Read the model definition and answer for the solid it produces. Units are mm, in the model's axes. A direction names the side the tool comes from. Give positions to 0.01 mm unless a question says otherwise; leave off trailing zeros. Write each loop counter-clockwise with the first axis right and the second up, starting at its lowest first coordinate (ties: lowest second). Pieces come first, ordered by that corner, then holes. Notation, with made-up numbers: (81.5, -16.5) - (118.5, -16.5) arc R26 ccw to (118.5, 8.5) - close; hole circle Ø8 at (82, 79.25). An arc over 180 degrees is marked (long way). Answer as CSV lines item,"result".
Autodesk Inventor part; units mm, degrees
ref_plane "YZ Plane" through (0, 0, 0) normal (1, 0, 0) x (0, 1, 0)
ref_plane "XZ Plane" through (0, 0, 0) normal (0, 1, 0) x (-1, 0, 0)
ref_plane "XY Plane" through (0, 0, 0) normal (0, 0, 1) x (1, 0, 0)
sketch "Szkic1" plane through (0, 0, 0) normal (0, 1, 0) x (-1, 0, 0)
  line L0 (8.460922, -2.595157) -> (8.460922, -202.595157)
  line L1 (8.460922, -202.595157) -> (-191.539078, -202.595157)
  line L2 (8.460922, -2.595157) -> (-191.539078, -2.595157)
  line L3 (8.460922, -2.595157) -> (208.460922, -2.595157) construction
  arc A0 (-191.539078, -2.595157) -> (-191.539078, -202.595157) centre (-145.713321, -102.595157) ccw
  line L4 (8.460922, -102.595157) -> (43.460922, -102.595157) construction
  circle A1 centre (-26.539078, -102.595157) radius 10
  point P0 (0, 0)
  dimension "d0" = 200
  dimension "d1" = 200
  dimension "d2" = 90
  dimension "d4" = 200
  dimension "d5" = 180
  dimension "d6" = 110
  dimension "d10" = 20
extrude "Wyciągnięcie proste1" add sketch "Szkic1" along normal blind 74.5
sketch "Szkic2" plane through (0, 74.5, 0) normal (0, 1, 0) x (1, 0, 0)
  circle A0 centre (107.96185, 52.890403) radius 34.51232
  circle A1 centre (113.959733, 99.782925) radius 48.14156
  point P0 (0, 0)
sketch "Szkic2 outline for Wyciągnięcie proste2" plane through (0, 74.5, 0) normal (0, 1, 0) x (1, 0, 0)
  circle A0 centre (113.959733, 99.782925) radius 48.14156
extrude "Wyciągnięcie proste2" add sketch "Szkic2 outline for Wyciągnięcie proste2" along normal blind 74.5 draft -10
hole "Otwór1" at (114.99325, 149, -100.1379) direction (0, -1, 0) diameter 25.75 end through all
(1) For faces 5 (the flat face through (90, 37, -202.595)), 6 (the flat face through (96, 74.5, -146)), determine the directions among +Z, -Z, +X, -X, +Y, -Y from which every point of the face is accessible in a straight line to the end or side of a thin tool.
Worked out:
face 5,"-Z, +X, -X, +Y, -Y"
face 6,"+Y"
(2) A cutting plane is placed at B-B (y = 80.5). Write down the section's boundary in (x, z) (3 decimals).
Worked out:
outline,"circle Ø94.167 at (113.96, -99.783); hole circle Ø25.75 at (114.993, -100.138)"
(3) Find the intervals of material crossed by L1, parallel to Y at x = 225.5, z = -138; L2, parallel to X at y = 30, z = -109.5; L3, parallel to Z at x = 123, y = 81.5, in increasing order.
Worked out:
L1,"y = 0 to 74.5"
L2,"x = -8.46 to 19.31, 33.77 to 106.15, 123.83 to 255.5"
L3,"z = -145.81 to -110.22, -90.06 to -53.76"
(4) A cutting plane is placed at D-D (z = -30). Write down the section's boundary in (x, y).
Worked out:
outline,"(-8.46, 0) - (228.36, 0) - (228.36, 74.5) - (-8.46, 74.5) - close"
(5) Each of these flat-tipped pins is pushed along its axis until it touches: P1, Ø10, axis at x = 182.5, z = -78.5, coming from the +Y side; P2, Ø12, axis at y = 27, z = -112.5, coming from the +X side; P3, Ø3, axis at x = 199.5, y = 34.5, coming from the -Z side. Where does it stop, or does it pass through?
Worked out:
P1,"stops at y = 74.5"
P2,"stops at x = 255.64"
P3,"stops at z = -199.37"
(6) A cutting plane is placed at A-A (x = 58). Write down the section's boundary in (y, z).
Worked out:
outline,"(0, -202.6) - (74.5, -202.6) - (74.5, -2.6) - (0, -2.6) - close"
(7) The mould has two halves that part along X. Classify faces 1 (the flat face through (129, 149, -100)), 2 (the cylindrical face through (17.3, 36.73, -98.77)), 3 (the cylindrical face through (106.292, 73.457, -109.627)), 4 (the flat face through (-8.461, 37, -101)): +X half, -X half, draft (parallel to the pull), parting line (faces both ways), or undercut.
Worked out:
face 1,"draft"
face 2,"undercut"
face 3,"undercut"
face 4,"-X half"
(8) A cutting plane is placed at C-C (y = 46.5). Write down the section's boundary in (x, z) (3 decimals).
Worked out:
outline,"(-8.461, -202.595) - (191.539, -202.595) arc R110 ccw to (191.539, -2.595) - (-8.461, -2.595) - close; hole circle Ø20 at (26.539, -102.595); hole circle Ø25.75 at (114.993, -100.138)"
